The listing builds one solid part. Answer for the finished solid, in the listing's coordinates (mm). Face numbers are marked on the shaded views. A direction names the side the tool comes from. Give positions to 0.01 mm unless a question says otherwise; leave off trailing zeros. Loops run counter-clockwise (first coordinate to the right, second up) from the corner with the lowest first, then second, coordinate; pieces in that order, holes last. Notation, with made-up numbers: (22.25, 49.5) - (62.25, 49.5) arc R22 ccw to (62.25, 60.5) - close; hole circle Ø4 at (89.25, 61.25). An arc over 180 degrees is marked (long way). Write each question's results on one line, items separated by ' | '.
from build123d import *

# Parameters (mm, degrees)
F0_W     = 40
F0_H     = 40
F1_DEPTH = 20
F3_DEPTH = 20
F6_DEPTH = 20


with BuildPart() as f1:
    # F0 (on Top) → F1 (new body, symmetric)
    with BuildSketch(Plane.XY):
        Rectangle(F0_W, F0_H)
    extrude(amount=F1_DEPTH, both=True)

    # F2 (on Top) → F3 (intersect, symmetric)
    with BuildSketch(Plane.XY):
        Polygon((20, 20), (-20, 20), (-20, 10), (-5, 10), (-5, -20), (5, -20), (5, 10), (20, 10), align=None)
    extrude(amount=F3_DEPTH, both=True, mode=Mode.INTERSECT)

    # F5 (on Front) → F6 (intersect, symmetric)
    with BuildSketch(Plane.XZ):
        with BuildLine():
            Line((15, 20), (-15, 20))
            ThreePointArc((-15, 20), (-18.535534, 18.535534), (-20, 15))
            Line((-20, 15), (-20, -15))
            ThreePointArc((-20, -15), (-18.535534, -18.535534), (-15, -20))
            Line((-15, -20), (15, -20))
            ThreePointArc((15, -20), (18.535534, -18.535534), (20, -15))
            Line((20, -15), (20, -5))
            ThreePointArc((20, -5), (18.535534, -1.464466), (15, 0))
            Line((15, 0), (-4.470152, 0))
            Line((-4.470152, 0), (-4.470152, -6.666667))
            Line((-4.470152, -6.666667), (10.365012, -6.666667))
            Line((10.365012, -6.666667), (10.365012, -8.333333))
            ThreePointArc((10.365012, -8.333333), (8.900546, -11.868867), (5.365012, -13.333333))
            Line((5.365012, -13.333333), (-7.16246, -13.333333))
            ThreePointArc((-7.16246, -13.333333), (-10.697994, -11.868867), (-12.16246, -8.333333))
            Line((-12.16246, -8.333333), (-12.16246, 8.333333))
            ThreePointArc((-12.16246, 8.333333), (-10.697994, 11.868867), (-7.16246, 13.333333))
            Line((-7.16246, 13.333333), (6.648352, 13.333333))
            ThreePointArc((6.648352, 13.333333), (10.183886, 11.868867), (11.648352, 8.333333))
            Line((11.648352, 8.333333), (11.648352, 6.666667))
            Line((11.648352, 6.666667), (20, 6.666667))
            Line((20, 6.666667), (20, 15))
            ThreePointArc((20, 15), (18.535534, 18.535534), (15, 20))
        make_face()
    extrude(amount=F6_DEPTH, both=True, mode=Mode.INTERSECT)


solid = f1.part
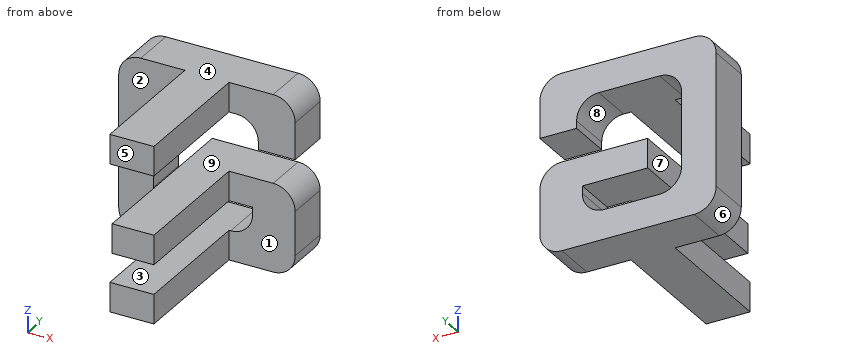
Item 1: A cutting plane is placed at D-D, the plane y = 13. Determine the outline of the cut face in (x, z), plus the area to 3 significant figures.
Values found:
outline: (-20, -15) arc R5 ccw to (-15, -20) - (15, -20) arc R5 ccw to (20, -15) - (20, -5) arc R5 ccw to (15, 0) - (-4.47, 0) - (-4.47, -6.67) - (10.37, -6.67) - (10.37, -8.33) arc R5 cw to (5.37, -13.33) - (-7.16, -13.33) arc R5 cw to (-12.16, -8.33) - (-12.16, 8.33) arc R5 cw to (-7.16, 13.33) - (6.65, 13.33) arc R5 cw to (11.65, 8.33) - (11.65, 6.67) - (20, 6.67) - (20, 15) arc R5 ccw to (15, 20) - (-15, 20) arc R5 ccw to (-20, 15) - close | area: 1,020 mm²
Item 2: Find the intervals of material crossed by line 1 along Z through (x, y) = (0, 7.5); line 2 along Z through (x, y) = (9, 16.5); line 3 along X through (y, z) = (18, 2), in increasing order. Write a range as [from, to].
Values found:
line 1: z = [-20, -13.33], [-6.67, 0], [13.33, 20] | line 2: z = [-20, -11.77], [-6.67, 0], [12.75, 20] | line 3: x = [-20, -12.16]
Item 3: Flat-ended cylindrical pins translate along their axes: P1, Ø4, axis at y = -13.5, z = -3, coming from the -X side; P2, Ø4, axis at y = -5, z = 13, coming from the +X side; P3, Ø7.5, axis at x = -16, z = -3.5, coming from the -Y side; P4, Ø1, axis at x = -9, y = 8, coming from the +Z side. Find the tip coordinate at first contact, or state that the pin passes through.
Values found:
P1: stops at x = -4.47 | P2: stops at x = 5 | P3: stops at y = 10 | P4: passes through
Item 4: A cutting plane is placed at A-A, the plane y = 5. Determine the outline of the cut face in (x, z).
Values found:
outline: (-5, -20) - (5, -20) - (5, -13.33) - (-5, -13.33) - close; (-5, 13.33) - (5, 13.33) - (5, 20) - (-5, 20) - close; (-4.47, -6.67) - (5, -6.67) - (5, 0) - (-4.47, 0) - close
Item 5: For the marked faces 1, 2, 3, 4 and 5, determine the directions among +Z, -Z, +X, -X, +Y, -Y from which every point of the face is accessible in a straight line to the end or side of a thin tool.
Values found:
face 1: +Z, -Z, +X, -Y | face 2: +Z, -Z, -X, -Y | face 3: +Y, -Y | face 4: +Z, +X, -X, +Y, -Y | face 5: +Z, -Z, +X, -X, -Y
Item 6: A cutting plane is placed at C-C, the plane x = -0.5. Determine the outline of the cut face in (y, z).
Values found:
outline: (-20, -20) - (20, -20) - (20, -13.33) - (-20, -13.33) - close; (-20, -6.67) - (20, -6.67) - (20, 0) - (-20, 0) - close; (-20, 13.33) - (20, 13.33) - (20, 20) - (-20, 20) - close
Item 7: For a pull along X with two mould halves and no side action, classify the marked faces 6, 7, 8 and 9 as released by +X, released by -X, zero draft, split by the parting line, or undercut.
Values found:
face 6: released by -X | face 7: undercut | face 8: undercut | face 9: zero draft
Item 8: A cutting plane is placed at B-B, the plane z = -7.5. Determine the outline of the cut face in (x, y), plus the area to 3 significant figures.
Values found:
outline: (-20, 10) - (-12.16, 10) - (-12.16, 20) - (-20, 20) - close; (10.37, 10) - (20, 10) - (20, 20) - (10.37, 20) - close | area: 175 mm²
